Source: CAD feature listing. Evaluate the final solid. Frame: model axes, mm. A direction names the side the tool comes from. Coordinates: 2 decimals unless noted, no trailing zeros. Write each loop counter-clockwise with the first axis right and the second up, starting at its lowest first coordinate (ties: lowest second). Pieces come first, ordered by that corner, then holes. Notation, with made-up numbers: M 57,43 L 69,43 A34 cw 69,73 Z; hole C -22.75,63 d2. An arc over 180 degrees is marked long. Write item = value, one per line. Start each with the question number.
1. Section query A-A (y = 24.5). Output: boundary loops of the cut face in (x, z).
2. Line query: line 1 along X through (y, z) = (22, 2.25); line 2 along Y through (x, z) = (181.5, 0.5). Output: solid intervals per line, ascending.
3. Section query C-C (x = 185). Output: boundary loops of the cut face in (y, z).
4. Section query B-B (z = 5). Output: boundary loops of the cut face in (x, y), then the cut area to 3 significant figures.
5. Access query for faces 1 (the face through (138, 50.8, 3)), 2 (the face through (88.9, 16, 3)). Directions: +Z, -Z, +X, -X, +Y, -Y. A direction counts if a zero-diameter tool reaches every point of the face in a straight line with its end or side. Return the directions, or none.
6. Pull-direction query (X, two-part tool) for faces 3 (the face through (0, 25, 3)), 4 (the face through (139, 31.75, 3)), 5 (the face through (138, 37, 0)); classes: pulls with the +X half, pulls with the -X half, needs draft (parallel to the pull), parting line crosses it, or undercut.
7. Pin query (flat end, axial travel): pin 1 Ø1.5 at (y, z) = (8.5, 2) entering from -X. Return the tip coordinate at first contact, or that it passes through.
```python
from build123d import *

# Parameters (mm, degrees)
BOX001_W                    = 279.4
BOX001_H                    = 50.8
BOX001_DEPTH                = 6.35
BOX001_PLACEMENT_ANGLE      = 30
BASEFEATURE_PLACEMENT_ANGLE = 30
SKETCH001_W                 = 101.6
SKETCH001_H                 = 31.75
POCKET_DEPTH                = 6.351


with BuildPart() as part:
    # Box001 → Box001 (new body)
    with BuildSketch(Plane.XY):
        with Locations((139.7, 25.4)):
            Rectangle(BOX001_W, BOX001_H)
    extrude(amount=BOX001_DEPTH)


with BuildPart() as part_1:
    # Box001 placement: moved
    add(part.part.moved(Location((0, 0, -417.576))).rotate(Axis((0, 0, -417.576), (-1, 0, 0)), BOX001_PLACEMENT_ANGLE))


with BuildPart() as part_2:
    # BaseFeature placement: moved
    add(part_1.part.moved(Location((0, -208.788, 361.631424))).rotate(Axis((0, -208.788, 361.631424), (1, 0, 0)), BASEFEATURE_PLACEMENT_ANGLE))

    # Sketch001 (on DatumPlane) → Pocket (cut, through all)
    with BuildSketch(Plane.XY.offset(6.35)):
        with Locations((139.7, 15.875)):
            Rectangle(SKETCH001_W, SKETCH001_H)
    extrude(amount=-POCKET_DEPTH, mode=Mode.SUBTRACT)


solid = part_2.part
```
Results are:
q1.outline = M 0,0 L 88.9,0 L 88.9,6.35 L 0,6.35 Z; M 190.5,0 L 279.4,0 L 279.4,6.35 L 190.5,6.35 Z
q2.line_1 = 0 to 88.9, 190.5 to 279.4
q2.line_2 = 31.75 to 50.8
q3.outline = M 31.75,0 L 50.8,0 L 50.8,6.35 L 31.75,6.35 Z
q4.outline = M 0,0 L 88.9,0 L 88.9,31.75 L 190.5,31.75 L 190.5,0 L 279.4,0 L 279.4,50.8 L 0,50.8 Z
q4.area = 11,000 mm^2
q5.face_1 = +Z, -Z, +X, -X, +Y
q5.face_2 = +Z, -Z, -Y
q6.face_3 = pulls with the -X half
q6.face_4 = undercut
q6.face_5 = needs draft
q7.pin_1 = 0
